CAD build for the part. Positions are in the model's coordinates, mm. A direction names the side the tool comes from. Give positions to 0.01 mm unless a question says otherwise; leave off trailing zeros. Write each loop counter-clockwise with the first axis right and the second up, starting at its lowest first coordinate (ties: lowest second). Pieces come first, ordered by that corner, then holes. Notation, with made-up numbers: (-9, -5) - (32, -5) arc R18 cw to (32, 2) - close; hole circle Ø5 at (-1.5, 6). An arc over 180 degrees is marked (long way). Answer as a JSON object with one key per item and string values.
from build123d import *

# Parameters (mm, degrees)
CROQUIS1_R                = 5
SALIENTE_EXTRUIR1_DEPTH   = 140
TALADRO_ROSCADO_M61_D     = 5
TALADRO_ROSCADO_M61_DEPTH = 17
TALADRO_ROSCADO_M61_TIP   = 1.502151548
TALADRO_ROSCADO_M62_D     = 5
TALADRO_ROSCADO_M62_DEPTH = 17
TALADRO_ROSCADO_M62_TIP   = 1.502151548
CHAFL_N1_SIZE             = 1


with BuildPart() as part:
    # Croquis1 → Saliente-Extruir1 (new, symmetric)
    with BuildSketch(Plane.XY):
        Circle(CROQUIS1_R)
    extrude(amount=SALIENTE_EXTRUIR1_DEPTH, both=True)

    # Taladro roscado M61
    with Locations(Plane.XY.offset(140)):
        with Locations((0, 0)):
            Hole(TALADRO_ROSCADO_M61_D / 2, depth=TALADRO_ROSCADO_M61_DEPTH)
            with Locations((0, 0, -(TALADRO_ROSCADO_M61_DEPTH + TALADRO_ROSCADO_M61_TIP / 2))):  # 118° drill point
                Cone(0, TALADRO_ROSCADO_M61_D / 2, TALADRO_ROSCADO_M61_TIP, mode=Mode.SUBTRACT)

    # Taladro roscado M62
    with Locations(Plane(origin=(0, 0, -140), x_dir=(-1, 0, 0), z_dir=(0, 0, -1))):
        with Locations((0, 0)):
            Hole(TALADRO_ROSCADO_M62_D / 2, depth=TALADRO_ROSCADO_M62_DEPTH)
            with Locations((0, 0, -(TALADRO_ROSCADO_M62_DEPTH + TALADRO_ROSCADO_M62_TIP / 2))):  # 118° drill point
                Cone(0, TALADRO_ROSCADO_M62_D / 2, TALADRO_ROSCADO_M62_TIP, mode=Mode.SUBTRACT)

    # Chaflán1
    chafl_n1_edges = [part.edges().sort_by_distance(p)[0] for p in [
        (-5, 0, -140),
    ]]
    chamfer(chafl_n1_edges, length=CHAFL_N1_SIZE)


solid = part.part
Item 1: Which spindle directions (+Z, -Z, +X, -X, +Y, -Y) get a long thin tool onto all of the face, cutting with end or side? Do faces 1 (the cylindrical face through (-0.54, -2.44, -131.38)), 2 (the flat face through (2, -2, 140)). Say none if no direction does.
Entries:
{"face 1": "-Z", "face 2": "+Z, +X, -X, +Y, -Y"}
Item 2: Cut at A-A (z = 75.5). Give the cut face in (x, y), and give its area (3 significant figures).
Entries:
{"outline": "circle Ø10 at (0, 0)", "area": "78.5 mm2"}
Item 3: Probe line 1 (Y direction, x = 0, z = -134.5); line 2 (Z direction, x = 0.25, y = 4); line 3 (X direction, y = 3, z = -111.5). List the from-to ranges inside material, lowest first. Write a range as from..to.
Entries:
{"line 1": "-5..-2.5, 2.5..5", "line 2": "-139.99..140", "line 3": "-4..4"}
Item 4: Mould opens along Y. For faces 3 (the flat face through (2, 2, -140)), 4 (the cylindrical face through (0.54, -2.44, 131.38)), 5 (the cylindrical face through (-1.08, -4.88, 2.45)) say: +Y half, -Y half, draft (parallel to the pull), parting line (faces both ways), or undercut.
Entries:
{"face 3": "draft", "face 4": "undercut", "face 5": "parting line"}
Item 5: Flat gauge pins, fed straight in: P1, Ø1.5, axis at x = 2, z = -9.5, coming from the +Y side; P2, Ø4, axis at y = 3, z = 77, coming from the -X side; P3, Ø4.5, axis at x = 0, y = 0, coming from the -Z side. Where does each tip first touch, or does it go through?
Entries:
{"P1": "y = 4.84", "P2": "x = -4.9", "P3": "z = -122.85"}
